Build history of the part. All positions in model axes, mm. A direction names the side the tool comes from. Give positions to 0.01 mm unless a question says otherwise; leave off trailing zeros. Loops run counter-clockwise (first coordinate to the right, second up) from the corner with the lowest first, then second, coordinate; pieces in that order, holes last. Notation, with made-up numbers: M 76,80.5 L 93,80.5 A10 ccw 93,94.5 Z; hole C 67.5,-5 d1. An arc over 180 degrees is marked long. Answer as a JSON object with one key per item and string values. Group by question number.
1. 3-axis set-ups, long thin cutter, end or side, ignore diameter. For faces 4 (the face through (5.45, 3.9, 29.99)), 5 (the face through (13, 33, 90)), 6 (the face through (7, 22, 75)), 7 (the face through (0, 34.7, 28)): which of +Z, -Z, +X, -X, +Y, -Y reach the whole face in a straight line?
2. Slice it at B-B (y = 11). List the corners of the cut face in (x, z).
3. Drop flat-ended pins along their axis: pin 1 Ø7.5 at (x, z) = (17.5, 53.5) entering from -Y; pin 2 Ø8 at (x, y) = (25, 10) entering from +Z; pin 3 Ø12 at (x, y) = (25.5, 9) entering from +Z. Give the stop position or say it passes through.
4. Slice it at A-A (z = 69). List the corners of the cut face in (x, y).
5. Slice it at C-C (x = 18). List the corners of the cut face in (y, z).
6. Mould opens along X. For faces 1 (the face through (-21, 7.7, 30)), 2 (the face through (10, 21.7, 55)), 3 (the face through (16.45, 21, -1)) say: released by +X, released by -X, zero draft, split by the parting line, or undercut.
7. Drill centre lines: line 1 along Z through (x, y) = (-10, 24.5) (3 decimals); line 2 along X through (y, z) = (27.5, 55) (3 decimals); line 3 along X through (y, z) = (28, 73). Where is each one in solid material? Low to high. Write a range as [from, to].
from build123d import *

# Parameters (mm, degrees)
BOSS_EXTRUDE1_DEPTH     = 7.7
SKETCH2_W               = 7
SKETCH2_H               = 3.1
CUT_EXTRUDE1_DEPTH      = 79.027559234
FILLET1_R               = 10
BOSS_EXTRUDE2_DEPTH     = 2
SKETCH4_W               = 109.5
SKETCH4_H               = 25
BOSS_EXTRUDE3_DEPTH     = 33.45
BOSS_EXTRUDE4_REACH     = 117.534
CUT_EXTRUDE2_DEPTH      = 114.458814113
CUT_EXTRUDE2_DEPTH_BACK = 114.458814113
CUT_EXTRUDE3_DEPTH      = 10
FILLET3_R               = 1
CUT_EXTRUDE5_REACH      = 117.534
SKETCH9_W               = 30
SKETCH9_H               = 4
FILLET5_R               = 3
CUT_EXTRUDE4_REACH      = 119.132
SKETCH8_W               = 17
SKETCH8_H               = 5
SKETCH8_W_2             = 19
SKETCH8_H_2             = 7
FILLET6_R               = 2
FILLET7_R               = 2
SKETCH11_W              = 10
SKETCH11_H              = 10
CUT_EXTRUDE6_DEPTH      = 22
CUT_EXTRUDE9_DEPTH      = 5
SKETCH12_R              = 2.275
CUT_EXTRUDE7_DEPTH      = 8
CHAMFER1_SIZE           = 0.5
SKETCH13_W              = 2
SKETCH13_H              = 9
SKETCH13_W_2            = 10
SKETCH13_H_2            = 6
CUT_EXTRUDE10_DEPTH     = 18


with BuildPart() as part:
    # Sketch1 → Boss-Extrude1 (new body)
    with BuildSketch(Plane(origin=(0, 0, 0), x_dir=(1, 0, 0), z_dir=(0, 1, 0))):
        Polygon((0, 0), (-16.35, 0), (-16.35, -9.85), (-2.6, -9.85), (-2.6, -33), (-20.1, -33), (-20.1, -75), (0, -75), align=None)
    extrude(amount=BOSS_EXTRUDE1_DEPTH)

    # Sketch2 → Cut-Extrude1 (cut, through all)
    with BuildSketch(Plane.XY.offset(75)):
        with Locations((-16.6, 3.55)):
            Rectangle(SKETCH2_W, SKETCH2_H)
    extrude(amount=-CUT_EXTRUDE1_DEPTH, mode=Mode.SUBTRACT)

    # Fillet1
    fillet1_edges = [part.edges().sort_by_distance(p)[0] for p in [
        (-2.6, 3.85, 33),
    ]]
    fillet(fillet1_edges, radius=FILLET1_R)

    # Sketch3 → Boss-Extrude2 (add)
    with BuildSketch(Plane(origin=(0, 7.7, 0), x_dir=(1, 0, 0), z_dir=(0, 1, 0))):
        Polygon((0, 4.5), (-33.45, 4.5), (-33.45, -75), (-10, -105), (0, -105), align=None)
    extrude(amount=BOSS_EXTRUDE2_DEPTH)

    # Sketch4 → Boss-Extrude3 (add)
    with BuildSketch(Plane(origin=(0, 0, 0), x_dir=(0, 0, -1), z_dir=(1, 0, 0))):
        with Locations((-50.25, 22.2)):
            Rectangle(SKETCH4_W, SKETCH4_H)
    extrude(amount=-BOSS_EXTRUDE3_DEPTH)

    # Boss-Extrude4: up to this face of the body (flat: up to its plane)
    boss_extrude4_end = Plane(part.part.faces().sort_by_distance((0, 18.36479202, 48.166489813))[0])
    # Sketch5 → Boss-Extrude4 (add, up to the picked face)
    with BuildSketch(Plane.ZY.offset(33.45), mode=Mode.PRIVATE) as boss_extrude4_sk1:
        Polygon((75, 7.7), (75, -5), (82, -5), (105, 7.7), align=None)
    boss_extrude4_tool1 = split(extrude(boss_extrude4_sk1.sketch, amount=-BOSS_EXTRUDE4_REACH, mode=Mode.PRIVATE), bisect_by=boss_extrude4_end, keep=Keep.BOTH, mode=Mode.PRIVATE)
    add(boss_extrude4_tool1.solids().sort_by(Axis((-33.45, 2.665766, 85.441441), (1, 0, 0)))[0])

    # Sketch6 → Cut-Extrude2 (cut, two sides: drawn at the far end of the back side and taken through both)
    with BuildSketch(Plane(origin=(0, 7.7, 0), x_dir=(1, 0, 0), z_dir=(0, 1, 0)).offset(-CUT_EXTRUDE2_DEPTH_BACK)):
        Polygon((-33.45, -75), (-10, -105), (-33.45, -105), align=None)
    extrude(amount=CUT_EXTRUDE2_DEPTH + CUT_EXTRUDE2_DEPTH_BACK, mode=Mode.SUBTRACT)

    # Sketch7 → Cut-Extrude3 (cut)
    with BuildSketch(Plane(origin=(0, 0, 0), x_dir=(0, 0, -1), z_dir=(1, 0, 0))):
        Polygon((-75, 0), (-85, 0), (-80, -5), (-75, -5), align=None)
    extrude(amount=-CUT_EXTRUDE3_DEPTH, mode=Mode.SUBTRACT)

    # Fillet3
    # the kernel refuses this fillet: 1 mm, written as the material it takes off along each edge
    with BuildSketch(Plane(origin=(5.810983209, -5, 80), x_dir=(0, 0.707106781186549, 0.7071067811865459), z_dir=(-1, 0, 0))) as fillet3_piece_1:
        with BuildLine():
            CenterArc((2.324393283, -1), FILLET3_R, 90, 114.469800521)
            Line((1.414213562, -1.414213562), (1.396009968, -1.422497834))
            ThreePointArc((1.396009968, -1.422497834), (0.692964646, -0.721248917), (-0.014142136, -0.014142136))
            Line((-0.014142136, -0.014142136), (0, 0.02))
            Line((0, 0.02), (2.324393283, 0.02))
            Line((2.324393283, 0.02), (2.324393283, 0))
        make_face()
    extrude(amount=15.810983209, mode=Mode.SUBTRACT)
    with BuildSketch(Plane(origin=(-10, -5, 82.5), x_dir=(0, 1, 0), z_dir=(0, 0, -1))) as fillet3_piece_2_section:
        with BuildLine():
            CenterArc((FILLET3_R, -FILLET3_R), FILLET3_R, 90, 90)
            Line((0, -FILLET3_R), (-FILLET3_R * 0.02, -FILLET3_R))
            Line((-FILLET3_R * 0.02, -FILLET3_R), (-FILLET3_R * 0.02, FILLET3_R * 0.02))
            Line((-FILLET3_R * 0.02, FILLET3_R * 0.02), (FILLET3_R, FILLET3_R * 0.02))
            Line((FILLET3_R, FILLET3_R * 0.02), (FILLET3_R, 0))
        make_face()
    fillet3_piece_2 = extrude(amount=10, mode=Mode.PRIVATE)
    fillet3_piece_2 = split(fillet3_piece_2, bisect_by=Plane(origin=(-10.222841489, -6.700692184, 78.299307816), z_dir=(0, 0.7071067811865466, -0.7071067811865485)), keep=Keep.TOP, mode=Mode.PRIVATE)
    add(fillet3_piece_2, mode=Mode.SUBTRACT)
    with BuildSketch(Plane(origin=(5.810983209, -5, 80), x_dir=(0, 0.707106781186549, 0.7071067811865459), z_dir=(-1, 0, 0))) as fillet3_piece_3a_section:
        with BuildLine():
            CenterArc((2.324393283, -1), FILLET3_R, 90, 114.469800521)
            Line((1.414213562, -1.414213562), (1.396009968, -1.422497834))
            ThreePointArc((1.396009968, -1.422497834), (0.692964646, -0.721248917), (-0.014142136, -0.014142136))
            Line((-0.014142136, -0.014142136), (0, 0.02))
            Line((0, 0.02), (2.324393283, 0.02))
            Line((2.324393283, 0.02), (2.324393283, 0))
        make_face()
    fillet3_piece_3a = extrude(amount=21.621966417, mode=Mode.PRIVATE)
    fillet3_piece_3a = split(fillet3_piece_3a, bisect_by=Plane(origin=(-10, -4.567151235, 80.996776665), z_dir=(-1, 0, 0)), keep=Keep.TOP, mode=Mode.PRIVATE)
    with BuildSketch(Plane(origin=(-10, -5, 82.5), x_dir=(0, 1, 0), z_dir=(0, 0, -1))) as fillet3_piece_3b_section:
        with BuildLine():
            CenterArc((FILLET3_R, -FILLET3_R), FILLET3_R, 90, 90)
            Line((0, -FILLET3_R), (-FILLET3_R * 0.02, -FILLET3_R))
            Line((-FILLET3_R * 0.02, -FILLET3_R), (-FILLET3_R * 0.02, FILLET3_R * 0.02))
            Line((-FILLET3_R * 0.02, FILLET3_R * 0.02), (FILLET3_R, FILLET3_R * 0.02))
            Line((FILLET3_R, FILLET3_R * 0.02), (FILLET3_R, 0))
        make_face()
    fillet3_piece_3b = extrude(amount=10, mode=Mode.PRIVATE)
    fillet3_piece_3b = split(fillet3_piece_3b, bisect_by=Plane(origin=(-10.238471404, -4.220535034, 80.779464966), z_dir=(0, -0.7071067811865466, 0.7071067811865485)), keep=Keep.TOP, mode=Mode.PRIVATE)
    fillet3_piece_3 = fillet3_piece_3a & fillet3_piece_3b
    add(fillet3_piece_3, mode=Mode.SUBTRACT)

    # Sketch9 → Cut-Extrude5 (cut, up to next)
    with BuildSketch(Plane(origin=(0, 0, 0), x_dir=(0, 0, -1), z_dir=(1, 0, 0)), mode=Mode.PRIVATE) as cut_extrude5_sk1:
        with Locations((-75, 32.7)):
            Rectangle(SKETCH9_W, SKETCH9_H)
    cut_extrude5_tool1 = extrude(cut_extrude5_sk1.sketch, amount=-CUT_EXTRUDE5_REACH, mode=Mode.PRIVATE) & part.part
    add(cut_extrude5_tool1.solids().sort_by_distance((0, 32.7, 75))[0], mode=Mode.SUBTRACT)

    # Mirror1: part across plane


with BuildPart() as part_1:
    add(part.part)
    add(part.part.mirror(Plane(origin=(0, 7.7, 75), x_dir=(0, 0, 1), z_dir=(-1, 0, 0))))

    # Fillet5
    # the kernel refuses this fillet: 3 mm, written as the material it takes off along each edge
    with BuildSketch(Plane(origin=(-38.068859068, -5, 69.091011854), x_dir=(0, 1, 0), z_dir=(0.6158478756904763, 0, 0.7878650861711843)), Plane(origin=(38.068859068, -5, 69.091011854), x_dir=(-0.7878650861711843, 0, -0.6158478756904764), z_dir=(-0.6158478756904763, 0, 0.7878650861711843))) as fillet5_piece_1:
        with BuildLine():
            CenterArc((FILLET5_R, -FILLET5_R), FILLET5_R, 90, 90)
            Line((0, -FILLET5_R), (0, 0))
            Line((0, 0), (FILLET5_R, 0))
        make_face()
    extrude(amount=23.884769896, mode=Mode.SUBTRACT)

    # Cut-Extrude4: up to this face of the body (flat: up to its plane)
    cut_extrude4_end = Plane(part_1.part.faces().sort_by_distance((0, 0, 47.459676899))[0])
    # Sketch8 → Cut-Extrude4 (cut, up to the picked face)
    with BuildSketch(Plane(origin=(0, 34.7, 0), x_dir=(1, 0, 0), z_dir=(0, 1, 0)), mode=Mode.PRIVATE) as cut_extrude4_sk1:
        with Locations((24.95, 2)):
            Rectangle(SKETCH8_W, SKETCH8_H)
    cut_extrude4_tool1 = split(extrude(cut_extrude4_sk1.sketch, amount=-CUT_EXTRUDE4_REACH, mode=Mode.PRIVATE), bisect_by=cut_extrude4_end, keep=Keep.BOTH, mode=Mode.PRIVATE)
    # Sketch8 → Cut-Extrude4 (cut, up to the picked face)
    with BuildSketch(Plane(origin=(0, 34.7, 0), x_dir=(1, 0, 0), z_dir=(0, 1, 0)), mode=Mode.PRIVATE) as cut_extrude4_sk2:
        with Locations((-24.95, 2)):
            Rectangle(SKETCH8_W_2, SKETCH8_H_2)
    cut_extrude4_tool2 = split(extrude(cut_extrude4_sk2.sketch, amount=-CUT_EXTRUDE4_REACH, mode=Mode.PRIVATE), bisect_by=cut_extrude4_end, keep=Keep.BOTH, mode=Mode.PRIVATE)
    add(cut_extrude4_tool1.solids().sort_by(Axis((24.95, 34.7, -2), (0, -1, 0)))[0], mode=Mode.SUBTRACT)
    add(cut_extrude4_tool2.solids().sort_by(Axis((-24.95, 34.7, -2), (0, -1, 0)))[0], mode=Mode.SUBTRACT)

    # Fillet6
    fillet6_edges = [part_1.edges().sort_by_distance(p)[0] for p in [
        (-15.45, 21.2, -4.5),
        (-33.45, 21.2, 1.5),
    ]]
    fillet(fillet6_edges, radius=FILLET6_R)

    # Fillet7
    fillet7_edges = [part_1.edges().sort_by_distance(p)[0] for p in [
        (33.45, 21.2, 0.5),
        (16.45, 21.2, -4.5),
    ]]
    fillet(fillet7_edges, radius=FILLET7_R)

    # Sketch11 → Cut-Extrude6 (cut)
    with BuildSketch(Plane(origin=(0, 34.7, 0), x_dir=(1, 0, 0), z_dir=(0, 1, 0))):
        Polygon((-5, -90), (-5, -100), (5, -100), (5, -60), (-5, -60), align=None)
        with Locations((0, -55)):
            Rectangle(SKETCH11_W, SKETCH11_H)
    extrude(amount=-CUT_EXTRUDE6_DEPTH, mode=Mode.SUBTRACT)

    # Sketch11<3> → Cut-Extrude9 (cut)
    with BuildSketch(Plane(origin=(0, 34.7, 0), x_dir=(1, 0, 0), z_dir=(0, 1, 0))):
        Polygon((-5, -90), (-5, -100), (5, -100), (5, -60), (5, -50), (-5, -50), align=None)
        with BuildLine():
            Line((-10, -100), (-5, -100))
            Line((-5, -100), (-5, -90))
            Line((-5, -90), (-15, -90))
            Line((-15, -90), (-15, -95))
            ThreePointArc((-15, -95), (-13.535533906, -98.535533906), (-10, -100))
        make_face()
        with BuildLine():
            Line((5, -50), (5, -60))
            Line((5, -60), (15, -60))
            Line((15, -60), (15, -55))
            ThreePointArc((15, -55), (13.535533906, -51.464466094), (10, -50))
            Line((10, -50), (5, -50))
        make_face()
    extrude(amount=-CUT_EXTRUDE9_DEPTH, mode=Mode.SUBTRACT)

    # Sketch12 → Cut-Extrude7 (cut)
    with BuildSketch(Plane(origin=(0, 29.7, 0), x_dir=(1, 0, 0), z_dir=(0, 1, 0))):
        with Locations(Location((10, -55, 0), (0, 0, 270))):
            Circle(SKETCH12_R)
        with Locations(Location((-10, -95, 0), (0, 0, 90))):
            Circle(SKETCH12_R)
    extrude(amount=-CUT_EXTRUDE7_DEPTH, mode=Mode.SUBTRACT)

    # Chamfer1
    chamfer1_edges = [part_1.edges().sort_by_distance(p)[0] for p in [
        (10, 29.7, 52.725),
        (-10, 29.7, 97.275),
    ]]
    chamfer(chamfer1_edges, length=CHAMFER1_SIZE)

    # Sketch13 → Cut-Extrude10 (cut)
    with BuildSketch(Plane(origin=(0, 30.7, 0), x_dir=(1, 0, 0), z_dir=(0, 1, 0))):
        with Locations((6, -75)):
            Rectangle(SKETCH13_W, SKETCH13_H)
        with Locations((-10, -75)):
            Rectangle(SKETCH13_W_2, SKETCH13_H_2)
    extrude(amount=-CUT_EXTRUDE10_DEPTH, mode=Mode.SUBTRACT)


solid = part_1.part
Established:
{
 "1": {"face 4": "+X, -Y", "face 5": "+X, -X, +Y", "face 6": "+Y", "face 7": "+Z, -Z, +X, -X, +Y"},
 "2": {"outline": "M -33.45,3.5 A2 ccw -31.45,1.5 L -15.45,1.5 L -15.45,-2.5 A2 ccw -13.45,-4.5 L 14.45,-4.5 A2 ccw 16.45,-2.5 L 16.45,0.5 L 31.45,0.5 A2 ccw 33.45,2.5 L 33.45,75 L 10,105 L -10,105 L -33.45,75 Z"},
 "3": {"pin 1": "stops at y = 0", "pin 2": "stops at z = 90.93", "pin 3": "stops at z = 92.85"},
 "4": {"outline": "M -33.45,7.7 L -20.1,7.7 L -20.1,5.1 L -13.1,5.1 L -13.1,2 L -20.1,2 L -20.1,0 L 20.1,0 L 20.1,2 L 13.1,2 L 13.1,5.1 L 20.1,5.1 L 20.1,7.7 L 33.45,7.7 L 33.45,30.7 L 5,30.7 L 5,12.7 L -5,12.7 L -5,30.7 L -33.45,30.7 Z"},
 "5": {"outline": "M -5,75 L 0,75 L 0,33 L 2,33 L 2,75 L 5.1,75 L 5.1,33 L 7.7,33 L 7.7,0.5 L 34.7,0.5 L 34.7,60 L 30.7,60 L 30.7,90 L 34.7,90 L 34.7,94.77 L 2.05,94.77 L -5,82 Z"},
 "6": {"face 1": "zero draft", "face 2": "undercut", "face 3": "released by +X"},
 "7": {"line 1": "z = [-4.5, 72], [78, 92.725], [97.275, 105]", "line 2": "x = [-33.45, -5], [5, 7.725], [12.275, 33.45]", "line 3": "x = [-33.45, -15], [7, 33.45]"}
}
